Here's how the part is built. I have some questions about the finished solid (model axes, mm). Face numbers are marked on the shaded views. A direction names the side the tool comes from. Coordinates: 2 decimals unless noted, no trailing zeros. Write each loop counter-clockwise with the first axis right and the second up, starting at its lowest first coordinate (ties: lowest second). Pieces come first, ordered by that corner, then holes.
Item 1: I want a section at D-D (x = 24.5). Please give me the cut outline in (y, z), and give its area (3 significant figures).
Item 2: I want a section at A-A (x = -45). Please give me the cut outline in (y, z).
Item 3: I want a section at B-B (y = 24). Please give me the cut outline in (x, z).
Item 4: For the marked faces 4, 5, 6 and 7, which set-ups out of +Z, -Z, +X, -X, +Y, -Y let a thin tool reach every point of the face, with its end or its side?
Item 5: If we mould it in two halves opening along Z, with no side actions, what happens to the marked faces 1, 2 and 3? For each: pulls with the +Z half, pulls with the -Z half, needs draft (parallel to the pull), parting line crosses it, or undercut.
Item 6: I'm going to push flat-ended pins straight in: P1, Ø5, axis at x = 23.5, z = 6.5, coming from the +Y side; P2, Ø2, axis at y = 62, z = 19, coming from the +X side; P3, Ø1.7, axis at x = 51.5, z = -21, coming from the +Y side. Where does each tip first touch, or does it pass through?
Item 7: Please list where these lines run through material, in increasing order: line 1 (Z direction, x = -45, y = 34); line 2 (X direction, y = 13.5, z = 2.5); line 3 (X direction, y = 35, z = 0.5).
Item 8: I want a section at C-C (z = 0). Please give me the cut outline in (x, y), and give its area (3 significant figures).
from build123d import *

# Parameters (mm, degrees)
EXTRUDE1_DEPTH     = 53
HOLE1_D            = 13
HOLE1_DEPTH        = 53
SKETCH5_R          = 4
CUT_EXTRUDE1_DEPTH = 4
SKETCH6_R          = 5.5
CUT_EXTRUDE2_DEPTH = 3
SKETCH7_R          = 2
CUT_EXTRUDE3_DEPTH = 33
CUT_EXTRUDE4_DEPTH = 5


with BuildPart() as part:
    # Sketch1 → Extrude1 (new body)
    with BuildSketch(Plane(origin=(0, 0, 0), x_dir=(1, 0, 0), z_dir=(0, 1, 0))):
        with BuildLine():
            Line((-48.427781283, 31), (48.427781283, 31))
            ThreePointArc((48.427781283, 31), (57.5, 0), (48.427781283, -31))
            Line((48.427781283, -31), (-48.427781283, -31))
            ThreePointArc((-48.427781283, -31), (-57.5, 0), (-48.427781283, 31))
        make_face()
    extrude(amount=EXTRUDE1_DEPTH)

    # Sketch2 → Revolve1 (revolve)
    with BuildSketch(Plane.XY, mode=Mode.PRIVATE) as revolve1_sk:
        Polygon((0, 91), (-11.25, 91), (-11.25, 75), (-31, 75), (-31, 53), (0, 53), align=None)
    revolve(revolve1_sk.sketch.rotate(Axis((0, 0, 0), (0, 1, 0)), 270), axis=Axis((0, 0, 0), (0, 1, 0)))  # turned: the seam where the file's is

    # Hole1
    with Locations(Plane(origin=(0, 53, 0), x_dir=(-1, 0, 0), z_dir=(0, 1, 0))):
        with Locations((45, 0), (-45, 0)):
            Hole(HOLE1_D / 2, depth=HOLE1_DEPTH)

    # Sketch5 → Cut-Extrude1 (cut)
    with BuildSketch(Plane.XZ):
        with Locations(Location((0, 0, 0), (0, 0, 270))):  # turned: the seam where the file's is
            Circle(SKETCH5_R)
    extrude(amount=-CUT_EXTRUDE1_DEPTH, mode=Mode.SUBTRACT)

    # Sketch6 → Cut-Extrude2 (cut)
    with BuildSketch(Plane.XZ):
        with Locations(Location((35, -15, 0), (0, 0, 270))):  # turned: the seam where the file's is
            Circle(SKETCH6_R)
    extrude(amount=-CUT_EXTRUDE2_DEPTH, mode=Mode.SUBTRACT)

    # Sketch7 → Cut-Extrude3 (cut)
    with BuildSketch(Plane.XZ.offset(-3)):
        with Locations(Location((35, -15, 0), (0, 0, 270))):  # turned: the seam where the file's is
            Circle(SKETCH7_R)
    extrude(amount=-CUT_EXTRUDE3_DEPTH, mode=Mode.SUBTRACT)

    # Sketch8 → Cut-Revolve1 (revolve, cut)
    with BuildSketch(Plane(origin=(0, 0, 0), x_dir=(0.920504853, 0, -0.390731128), z_dir=(0.390731128, 0, 0.920504853)), mode=Mode.PRIVATE) as cut_revolve1_sk:
        Polygon((57.5, 28), (55, 28), (55, 33.4215), (53.517364509, 34.2775), (35, 34.2775), (35, 40), (57.5, 40), align=None)
    revolve(cut_revolve1_sk.sketch.rotate(Axis((47.484793311, 40, -20.156098913), (-0.920504853, 0, 0.390731128)), 270), axis=Axis((47.484793311, 40, -20.156098913), (-0.920504853, 0, 0.390731128)), mode=Mode.SUBTRACT)  # turned: the seam where the file's is

    # Sketch9 → Revolve2 (revolve)
    with BuildSketch(Plane(origin=(0, 0, 0), x_dir=(0.920504853, 0, -0.390731128), z_dir=(0.390731128, 0, 0.920504853)), mode=Mode.PRIVATE) as revolve2_sk:
        Polygon((55, 31), (55, 34.2775), (46, 34.2775), (45, 35.2775), (45, 40), (60, 40), (60, 31), align=None)
    revolve(revolve2_sk.sketch.rotate(Axis((68.658528533, 40, -29.14381628), (-0.920504853, 0, 0.390731128)), 270), axis=Axis((68.658528533, 40, -29.14381628), (-0.920504853, 0, 0.390731128)))  # turned: the seam where the file's is

    # Sketch10 → Cut-Extrude4 (cut)
    with BuildSketch(Plane(origin=(55.230291207, 0, -23.443867709), x_dir=(-0.390731128, 0, -0.920504853), z_dir=(0.920504853, 0, -0.390731128))):
        Polygon((4.041451884, 40), (2.020725942, 43.5), (-2.020725942, 43.5), (-4.041451884, 40), (-2.020725942, 36.5), (2.020725942, 36.5), align=None)
    extrude(amount=-CUT_EXTRUDE4_DEPTH, mode=Mode.SUBTRACT)


solid = part.part
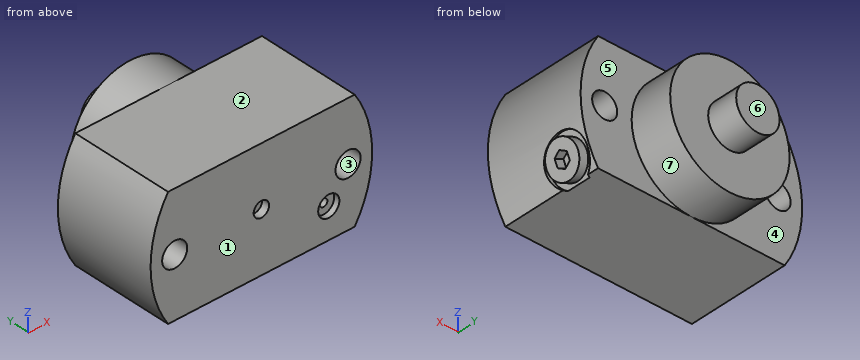
Answer:
1. outline: (0, -31) - (53, -31) - (53, -18.99) - (75, -18.99) - (75, 18.99) - (53, 18.99) - (53, 31) - (0, 31) - close
1. area: 4,120 mm2
2. outline: (0, -31) - (53, -31) - (53, -6.5) - (0, -6.5) - close; (0, 6.5) - (53, 6.5) - (53, 31) - (0, 31) - close
3. outline: (-48.43, -31) - (48.43, -31) arc R57.5 ccw to (48.43, 31) - (-48.43, 31) arc R57.5 ccw to start; hole circle Ø13 at (-45, 0); hole circle Ø4 at (35, -15); hole circle Ø13 at (45, 0)
4. face 4: -X, +Y
4. face 5: +X, +Y
4. face 6: +Z, -Z, +X, -X, +Y
4. face 7: +Y
5. face 1: needs draft
5. face 2: pulls with the +Z half
5. face 3: undercut
6. P1: stops at y = 75
6. P2: stops at x = 25.24
6. P3: stops at y = 53
7. line 1: z = -31 to -6.5, 6.5 to 31
7. line 2: x = -57.45 to -51, -39 to 39, 51 to 57.45
7. line 3: x = -57.5 to -51.48, -38.52 to 38.52, 51.48 to 57.5
8. outline: (-57.5, 0) - (-51.5, 0) - (-51.5, 53) - (-57.5, 53) - close; (-38.5, 0) - (-4, 0) - (-4, 4) - (4, 4) - (4, 0) - (38.5, 0) - (38.5, 53) - (31, 53) - (31, 75) - (11.25, 75) - (11.25, 91) - (-11.25, 91) - (-11.25, 75) - (-31, 75) - (-31, 53) - (-38.5, 53) - close; (51.5, 0) - (57.5, 0) - (57.5, 53) - (51.5, 53) - close
8. area: 6,410 mm2
